Input: dimensioned drawing with shaded views. Units: mm. Origin: part minimum x, y, z. A direction names the side the tool comes from. Give positions to 0.01 mm unless a question says otherwise; leave off trailing zeros. Write each loop counter-clockwise with the first axis right and the second up, starting at its lowest first coordinate (ties: lowest second). Pieces come first, ordered by that corner, then holes.
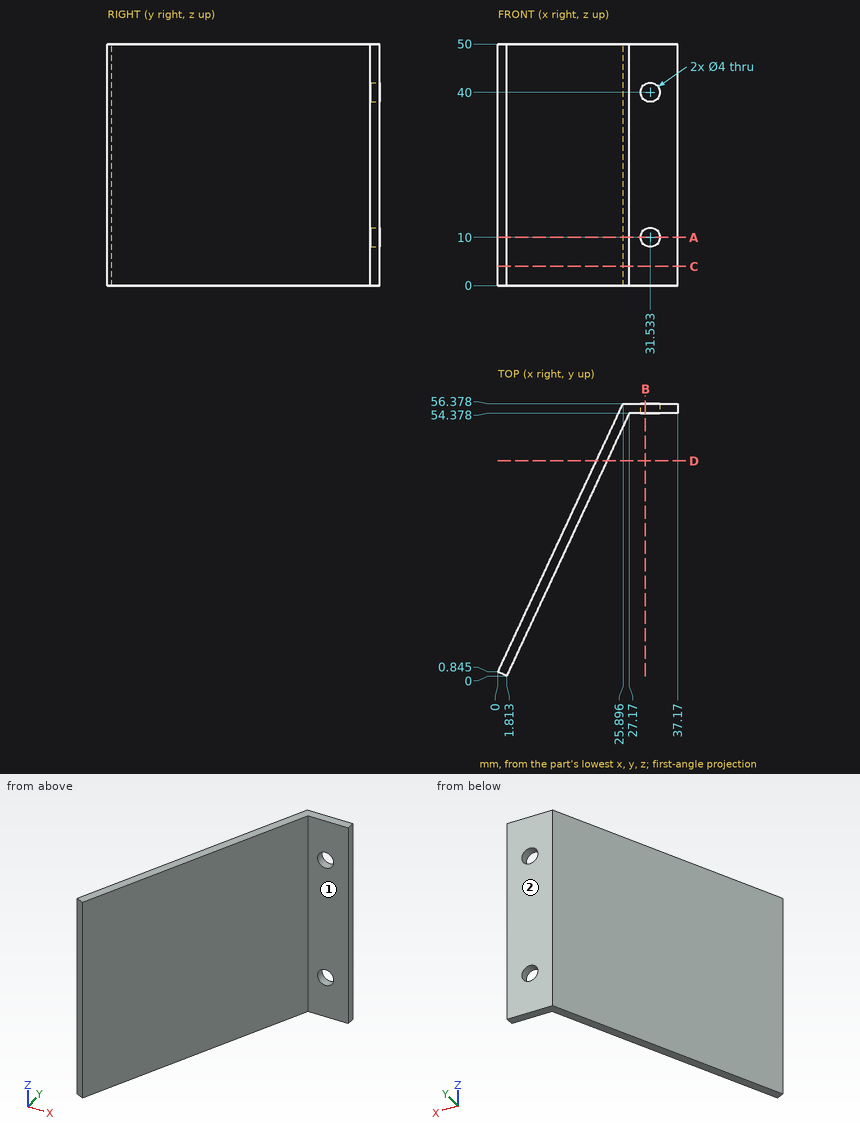
Item 1: Section D-D, the plane y = 44.5. Return the cut outline in (x, z), plus the area to 3 significant figures.
Found:
outline: (20.36, 0) - (22.56, 0) - (22.56, 50) - (20.36, 50) - close
area: 110 mm2
Item 2: Section C-C, the plane z = 4. Return the cut outline in (x, y) (1 decimal).
Found:
outline: (0, 0.8) - (1.8, 0) - (27.2, 54.4) - (37.2, 54.4) - (37.2, 56.4) - (25.9, 56.4) - close
Item 3: Line query: L1, parallel to X at y = 55.8, z = 10 (1 decimal); L2, parallel to Y at x = 32, z = 25; L3, parallel to X at y = 55.95, z = 10 (1 decimal). Output: solid intervals per line, ascending.
Found:
L1: x = 25.6 to 29.5, 33.5 to 37.2
L2: y = 54.38 to 56.38
L3: x = 25.7 to 29.5, 33.5 to 37.2
Item 4: Reachability of the marked faces 1 and 2 from +Z, -Z, +X, -X, +Y, -Y: full face, straight path, thin tool, end or side. Return the list, or none.
Found:
face 1: +Z, -Z, +X, -Y
face 2: +Z, -Z, +X, -X, +Y
Item 5: Section B-B, the plane x = 30.5. Return the cut outline in (y, z).
Found:
outline: (54.38, 0) - (56.38, 0) - (56.38, 8.29) - (54.38, 8.29) - close; (54.38, 11.71) - (56.38, 11.71) - (56.38, 38.29) - (54.38, 38.29) - close; (54.38, 41.71) - (56.38, 41.71) - (56.38, 50) - (54.38, 50) - close
Item 6: Pin query (flat end, axial travel): pin 1 Ø2.5 at (x, z) = (31.53, 10) entering from -Y; pin 2 Ø11 at (x, z) = (32.5, 25.5) entering from -Y (1 decimal); pin 3 Ø1.5 at (y, z) = (47.5, 14.5) entering from -X (1 decimal); pin 4 Ø1 at (y, z) = (10.5, 32.5) entering from -X. Return the tip coordinate at first contact, or that it passes through.
Found:
pin 1: passes through
pin 2: stops at y = 54
pin 3: stops at x = 21.4
pin 4: stops at x = 4.27
Item 7: Section A-A, the plane z = 10. Return the cut outline in (x, y) (1 decimal).
Found:
outline: (0, 0.8) - (1.8, 0) - (27.2, 54.4) - (29.5, 54.4) - (29.5, 56.4) - (25.9, 56.4) - close; (33.5, 54.4) - (37.2, 54.4) - (37.2, 56.4) - (33.5, 56.4) - close
